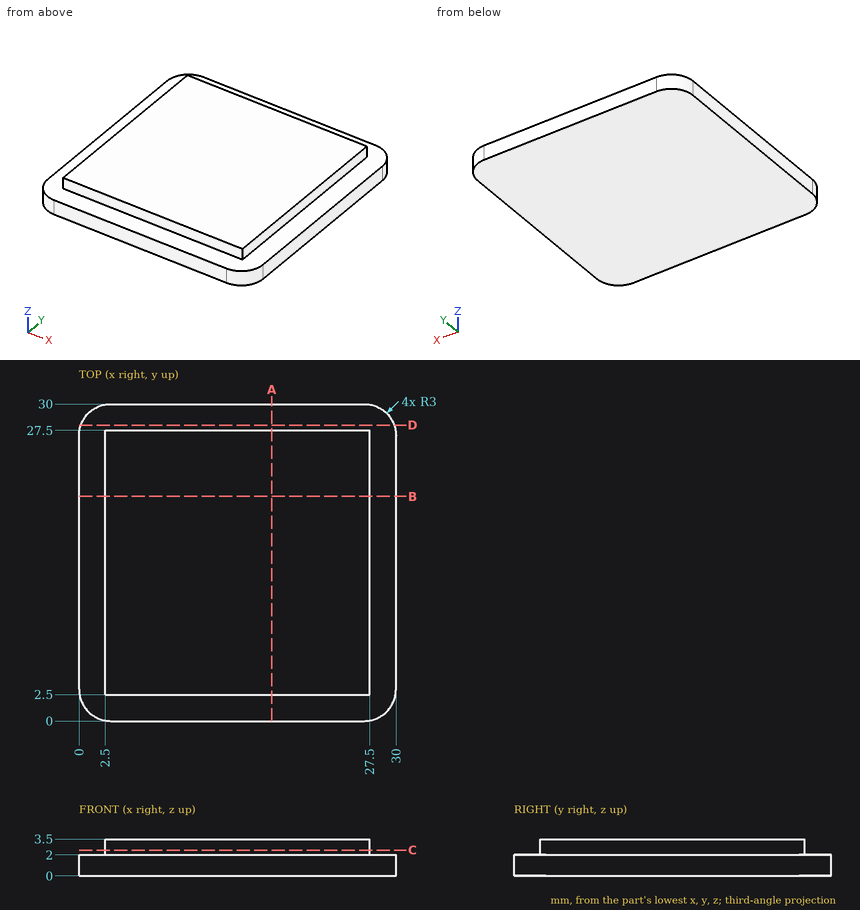
Design review of the part shown in the three views and the two pictorial views. Dimensions are in mm from the part's minimum x, y and z. Round coordinates to 2 decimals unless told otherwise and drop trailing zeros. Write each loop counter-clockwise with the first axis right and the second up, starting at its lowest first coordinate (ties: lowest second). Pieces come first, ordered by that corner, then holes. Notation, with made-up numbers: (-11, 31.5) - (40, 31.5) arc R14 cw to (40, 58.5) - close; hole circle Ø1 at (41.5, -7). An arc over 180 degrees is marked (long way). Write item = value, one per line. Start each with the question number.
1. Consider section D-D on y = 28. State the section outline as (x, z) points, plus the area to 3 significant figures.
2. Wall thickness on L1, parallel to X at y = 5.5, z = 3.3; L2, parallel to X at y = 27.75, z = 0.3: over which ranges is each line inside the solid? List them lowest first.
3. Consider section A-A on x = 18.25. State the section outline as (y, z) points, plus the area to 3 significant figures.
4. For pin 1 Ø1.2 at (x, z) = (18.5, 3) entering from +Y; pin 2 Ø1.6 at (x, z) = (17, 2.5) entering from -Y; pin 3 Ø0.8 at (y, z) = (15.5, 3) entering from +X, all flat-tipped, find the tip position at first contact; note any pin that passes through.
5. Consider section C-C on z = 2.45. State the section outline as (x, y) points.
Evaluation:
q1.outline = (0.17, 0) - (29.83, 0) - (29.83, 2) - (0.17, 2) - close
q1.area = 59.3 mm2
q2.L1 = 2.5 to 27.5
q2.L2 = 0.1 to 29.9
q3.outline = (0, 0) - (30, 0) - (30, 2) - (27.5, 2) - (27.5, 3.5) - (2.5, 3.5) - (2.5, 2) - (0, 2) - close
q3.area = 97.5 mm2
q4.pin_1 = 27.5
q4.pin_2 = 0
q4.pin_3 = 27.5
q5.outline = (2.5, 2.5) - (27.5, 2.5) - (27.5, 27.5) - (2.5, 27.5) - close
